from build123d import *

# Parameters (mm, degrees)
F0_W           = 5.7
F0_H           = 5
F1_DEPTH       = 2.75
F2_R           = 1.25
F2_R_2         = 0.585
F3_DEPTH       = 0.23
F4_DEPTH       = 3.12
F6_DEPTH       = 1.1
F7_R           = 0.45
F8_DEPTH       = 0.37
F10_DEPTH      = 2.2
F10_DEPTH_BACK = 2.2
F11_W          = 1.42
F11_H          = 2.75
F12_DEPTH      = 1.3
F12_DEPTH_BACK = 1.3


with BuildPart() as f1:
    # F0 (on Top) → F1 (new body)
    with BuildSketch(Plane.XY):
        with Locations((0.35, 0)):
            Rectangle(F0_W, F0_H)
    extrude(amount=-F1_DEPTH)

    # F2 (on face) → F3 (join)
    with BuildSketch(Plane.XY):
        Circle(F2_R)
        Circle(F2_R_2, mode=Mode.SUBTRACT)
    extrude(amount=F3_DEPTH)

    # F4 (add): a face of the model
    f4_faces = [f1.faces().sort_by_distance(p)[0] for p in [
        (0, 0, 0),
    ]]
    extrude(f4_faces, amount=F4_DEPTH)

    # F5 (on face) → F6 (cut)
    with BuildSketch(Plane.XY.offset(3.12)):
        with BuildLine():
            ThreePointArc((0.115, -0.573585216), (0.585, 0), (0.115, 0.573585216))
            Line((0.115, 0.573585216), (0.115, -0.573585216))
        make_face()
    extrude(amount=-F6_DEPTH, mode=Mode.SUBTRACT)

    # F7 (on face) → F8 (join)
    with BuildSketch(Plane(origin=(0, 0, -2.75), x_dir=(1, 0, 0), z_dir=(0, 0, -1))):
        with Locations((2.635, 1.8)):
            Circle(F7_R)
        with Locations((-1.935, 1.8)):
            Circle(F7_R)
        with Locations((-1.935, -1.8)):
            Circle(F7_R)
        with Locations((2.635, -1.8)):
            Circle(F7_R)
    extrude(amount=F8_DEPTH)

    # F9 (on Front) → F10 (join, two sides)
    with BuildSketch(Plane.XZ) as f10_sk:
        Polygon((3.6556336897, 0), (3.2, 0), (3.2, -0.25), (3.4802363597, -0.25), (4.3849187925, -2.75), (4.62, -2.6649304645), align=None)
    extrude(amount=F10_DEPTH)
    extrude(f10_sk.sketch, amount=-F10_DEPTH_BACK)

    # F11 (on Front) → F12 (cut, two sides)
    with BuildSketch(Plane.XZ) as f12_sk:
        with Locations((3.91, -1.375)):
            Rectangle(F11_W, F11_H)
    extrude(amount=-F12_DEPTH, mode=Mode.SUBTRACT)
    extrude(f12_sk.sketch, amount=F12_DEPTH_BACK, mode=Mode.SUBTRACT)


solid = f1.part
Source: CAD feature listing. Evaluate the final solid. Frame: model axes, mm. A direction names the side the tool comes from. Coordinates: 2 decimals unless noted, no trailing zeros. Loops run counter-clockwise (first coordinate to the right, second up) from the corner with the lowest first, then second, coordinate; pieces in that order, holes last. Notation, with made-up numbers: (15, -27.5) - (44, -27.5) arc R16 cw to (44, -1.5) - close; hole circle Ø3 at (9.25, -36.5). An arc over 180 degrees is marked (long way). One line per item, written item: value. Start each with the question number.
1. Mould query, pull axis X, two halves, no side actions, for faces 6 (the flat face through (0.115, 0, 2.6)), 7 (the flat face through (3.926, -1.756, -1.483)), 8 (the flat face through (0, -2.5, -1)). Classes: pulls with the +X half, pulls with the -X half, needs draft (parallel to the pull), parting line crosses it, or undercut.
2. Section C-C (z = -2). Return the cut outline in (x, y).
3. Set-up query: faces 1 (the flat face through (2.6, -1.8, -3.12)), 2 (the flat face through (0, -1, 0.23)), 3 (the cylindrical face through (2.877, -2.179, -2.932)), 4 (the flat face through (4.145, -1.756, -1.351)), 5 (the flat face through (3.926, 1.744, -1.483)). Return all of +Z, -Z, +X, -X, +Y, -Y with unobstructed straight access to the full face (end or side cutting, diameter ignored); none if empty.
4. Section A-A (y = 0). Return the cut outline in (x, z) (3 decimals), and give its area (3 significant figures).
5. Contact query for flat-ended pins moving along their axis: P1, Ø1.1, axis at x = 4, z = -1.5, coming from the +Y side; P2, Ø1, axis at x = 2.5, y = -1, coming from the -Z side; P3, Ø2, axis at x = 4, y = -1.5, coming from the +Z side; P4, Ø2, axis at y = 0, z = -2, coming from the +X side. Output: stop coordinate, or through.
6. Ray query, L1, parallel to Z at x = 3, y = -0.4; L2, parallel to X at y = 0.3, z = -0.25; L3, parallel to Z at x = 0.5, y = -0.65. Return the intervals inside material, ascending.
7. Section B-B (x = -1). Return the cut outline in (y, z), and give its area (3 significant figures).
8. Section D-D (y = 1.8). Return the cut outline in (x, z) (3 decimals).
Verdict:
1. face 6: pulls with the +X half
1. face 7: undercut
1. face 8: needs draft
2. outline: (-2.5, -2.5) - (3.2, -2.5) - (3.2, 2.5) - (-2.5, 2.5) - close; (4.11, -2.2) - (4.38, -2.2) - (4.38, -1.3) - (4.11, -1.3) - close; (4.11, 1.3) - (4.38, 1.3) - (4.38, 2.2) - (4.11, 2.2) - close
3. face 1: -Z, +X, -X, +Y, -Y
3. face 2: +Z
3. face 3: -Z
3. face 4: +Z, +X, +Y, -Y
3. face 5: -Z, +Y, -Y
4. outline: (-2.5, -2.75) - (3.2, -2.75) - (3.2, 0) - (1.25, 0) - (1.25, 0.23) - (0.585, 0.23) - (0.585, 2.02) - (0.115, 2.02) - (0.115, 3.12) - (-0.585, 3.12) - (-0.585, 0.23) - (-1.25, 0.23) - (-1.25, 0) - (-2.5, 0) - close
4. area: 19.1 mm2
5. P1: stops at y = 2.2
5. P2: stops at z = -3.12
5. P3: stops at z = 0
5. P4: stops at x = 3.2
6. L1: z = -2.75 to 0
6. L2: x = -2.5 to 3.2
6. L3: z = -2.75 to 0.23
7. outline: (-2.5, -2.75) - (2.5, -2.75) - (2.5, 0) - (0.75, 0) - (0.75, 0.23) - (-0.75, 0.23) - (-0.75, 0) - (-2.5, 0) - close
7. area: 14.1 mm2
8. outline: (-2.5, -2.75) - (-2.385, -2.75) - (-2.385, -3.12) - (-1.485, -3.12) - (-1.485, -2.75) - (2.185, -2.75) - (2.185, -3.12) - (3.085, -3.12) - (3.085, -2.75) - (3.2, -2.75) - (3.2, -0.25) - (3.48, -0.25) - (4.385, -2.75) - (4.62, -2.665) - (3.656, 0) - (-2.5, 0) - close
